Check sheet for the modelled part. Datum: model origin and axes. Units: mm. Give positions to 0.01 mm unless a question says otherwise; leave off trailing zeros. Order: outer loops, then holes, each group sorted by start corner. A loop starts at its lowest first (then second) coordinate and runs counter-clockwise, first axis right, second up.
Item 1: Sectioned sample at B-B on x = -9.5. Record the boundary of the cut face in (y, z), and give its area (3 significant figures).
Item 2: Sectioned sample at A-A on y = 0. Record the boundary of the cut face in (x, z).
Item 3: Gauge pin test, flat ends, axial feed: P1, Ø1.8, axis at x = 9.5, y = 0, coming from the +Z side; P2, Ø6.5, axis at x = 0, y = 23, coming from the +Z side. Record the tip position at first contact, or that the pin passes through.
Item 4: Sectioned sample at D-D on y = 23. Record the boundary of the cut face in (x, z), and give its area (3 significant figures).
Item 5: Sectioned sample at C-C on z = 0.85. Record the boundary of the cut face in (x, y).
Item 6: Material ranges on line 1 along Y through (x, z) = (0, 0.6); line 2 along Y through (x, z) = (-9.5, 0.85); line 3 along Y through (x, z) = (0.5, 0.85), recorded low to high.
from build123d import *

# Parameters (mm, degrees)
SKETCH1_W           = 30
SKETCH1_H           = 30
SKETCH1_R           = 4.25
SKETCH1_R_2         = 1.5
BOSS_EXTRUDE1_DEPTH = 2
SKETCH2_W           = 30
SKETCH2_H           = 2
BOSS_EXTRUDE2_DEPTH = 25
SKETCH3_R           = 2.5
CUT_EXTRUDE1_DEPTH  = 2


with BuildPart() as part:
    # Sketch1 → Boss-Extrude1 (new body)
    with BuildSketch(Plane.XY):
        Rectangle(SKETCH1_W, SKETCH1_H)
        Circle(SKETCH1_R, mode=Mode.SUBTRACT)
        with Locations((0, 9.5)):
            Circle(SKETCH1_R_2, mode=Mode.SUBTRACT)
        with Locations((9.5, 0)):
            Circle(SKETCH1_R_2, mode=Mode.SUBTRACT)
        with Locations((0, -9.5)):
            Circle(SKETCH1_R_2, mode=Mode.SUBTRACT)
        with Locations((-9.5, 0)):
            Circle(SKETCH1_R_2, mode=Mode.SUBTRACT)
    extrude(amount=BOSS_EXTRUDE1_DEPTH)

    # Sketch2 → Boss-Extrude2 (add)
    with BuildSketch(Plane(origin=(0, 15, 0), x_dir=(1, 0, 0), z_dir=(0, 1, 0))):
        with Locations((0, -1)):
            Rectangle(SKETCH2_W, SKETCH2_H)
    extrude(amount=BOSS_EXTRUDE2_DEPTH)

    # Sketch3 → Cut-Extrude1 (cut)
    with BuildSketch(Plane.XY.offset(2)):
        with Locations((0, 23)):
            Circle(SKETCH3_R)
        with Locations((0, 35)):
            Circle(SKETCH3_R)
    extrude(amount=-CUT_EXTRUDE1_DEPTH, mode=Mode.SUBTRACT)


solid = part.part
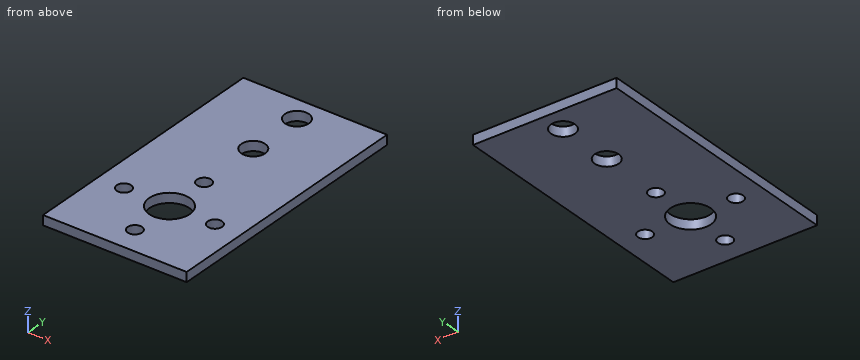
Report:
1. outline: (-15, 0) - (-1.5, 0) - (-1.5, 2) - (-15, 2) - close; (1.5, 0) - (40, 0) - (40, 2) - (1.5, 2) - close
1. area: 104 mm2
2. outline: (-15, 0) - (-11, 0) - (-11, 2) - (-15, 2) - close; (-8, 0) - (-4.25, 0) - (-4.25, 2) - (-8, 2) - close; (4.25, 0) - (8, 0) - (8, 2) - (4.25, 2) - close; (11, 0) - (15, 0) - (15, 2) - (11, 2) - close
3. P1: passes through
3. P2: stops at z = 2
4. outline: (-15, 0) - (-2.5, 0) - (-2.5, 2) - (-15, 2) - close; (2.5, 0) - (15, 0) - (15, 2) - (2.5, 2) - close
4. area: 50.0 mm2
5. outline: (-15, -15) - (15, -15) - (15, 40) - (-15, 40) - close; hole circle Ø3 at (-9.5, 0); hole circle Ø8.5 at (0, 0); hole circle Ø5 at (0, 23); hole circle Ø5 at (0, 35); hole circle Ø3 at (0, -9.5); hole circle Ø3 at (0, 9.5); hole circle Ø3 at (9.5, 0)
6. line 1: y = -15 to -11, -8 to -4.25, 4.25 to 8, 11 to 20.5, 25.5 to 32.5, 37.5 to 40
6. line 2: y = -15 to -1.5, 1.5 to 40
6. line 3: y = -15 to -10.91, -8.09 to -4.22, 4.22 to 8.09, 10.91 to 20.55, 25.45 to 32.55, 37.45 to 40
